Autodesk Inventor part; units mm, degrees
ref_plane "YZ Plane" through (0, 0, 0) normal (1, 0, 0) x (0, 1, 0)
ref_plane "XZ Plane" through (0, 0, 0) normal (0, 1, 0) x (-1, 0, 0)
ref_plane "XY Plane" through (0, 0, 0) normal (0, 0, 1) x (1, 0, 0)
sketch "Sketch1" plane through (0, 0, 0) normal (0, 0, 1) x (1, 0, 0)
  line L0 (-79.375, 79.375) -> (79.375, 79.375)
  line L1 (79.375, 79.375) -> (79.375, -79.375)
  line L2 (79.375, -79.375) -> (-79.375, -79.375)
  line L3 (-79.375, -79.375) -> (-79.375, 79.375)
  line L4 (-79.375, 79.375) -> (79.375, -79.375) construction
  line L5 (79.375, 79.375) -> (-79.375, -79.375) construction
  point P0 (0, 0)
  dimension "d0" = 158.75
extrude "Extrusion1" add sketch "Sketch1" along normal blind 50.8
shell "Shell1" thickness 3.175 outward yes removed faces 1 at (-26.4583, 26.4583, 50.8)
sketch "Sketch2" plane through (0, 0, 0) normal (0, 0, 1) x (1, 0, 0)
  line L0 (-82.55, 82.55) -> (-82.55, -82.55)
  circle A0 centre (-82.55, 82.55) radius 4.7752
  line L1 (82.55, -82.55) -> (82.55, 82.55)
  circle A1 centre (82.55, 82.55) radius 4.7752
  line L2 (-82.55, -82.55) -> (82.55, -82.55)
  circle A2 centre (82.55, -82.55) radius 4.7752
  circle A3 centre (-82.55, -82.55) radius 4.7752
  point P0 (0, 0)
  dimension "d4" = 9.5504
extrude "Extrusion2" add sketch "Sketch2" along normal blind 50.8 and the other way blind 3.175
sketch "Sketch3" plane through (0, 0, 50.8) normal (0, 0, 1) x (1, 0, 0)
  line L0 (-82.55, 77.7748) -> (-82.55, -77.7748)
  circle A0 centre (-82.55, -82.55) radius 1.7996
  circle A1 centre (82.55, 82.55) radius 1.7996
  line L1 (-77.7748, -82.55) -> (77.7748, -82.55)
  circle A2 centre (82.55, -82.55) radius 1.7996
  circle A3 centre (-82.55, 82.55) radius 1.7996
  point P0 (0, 0)
  dimension "d9" = 3.5992
extrude "Extrusion3" cut sketch "Sketch3" along normal mid plane 107.95
sketch "Sketch4" plane through (-77.7748, 82.55, -3.175) normal (0, 1, 0) x (1, 0, 0)
  line L0 (58.7248, -19.939) -> (96.8248, -19.939)
  line L1 (96.8248, -19.939) -> (96.8248, -42.545)
  line L2 (96.8248, -42.545) -> (58.7248, -42.545)
  line L3 (58.7248, -42.545) -> (58.7248, -19.939)
  line L4 (58.7248, -19.939) -> (96.8248, -42.545) construction
  line L5 (96.8248, -19.939) -> (58.7248, -42.545) construction
  line L6 (155.5496, -53.975) -> (0, -53.975)
  point P0 (77.7748, -3.175)
  point P1 (77.7748, -31.242)
  point P2 (77.7748, -31.242)
  point P3 (160.9128, -53.975)
  point P4 (-0.588, -53.975)
  dimension "d12" = 38.1
  dimension "d13" = 22.606
  dimension "d14" = 11.43
extrude "Extrusion4" cut sketch "Sketch4" against normal up to next
properties part number "PS-01" material "Aluminum 6061(1)"
Part model, mm, in its own coordinate system. A direction names the side the tool comes from. Coordinates: 2 decimals unless noted, no trailing zeros. Order: outer loops, then holes, each group sorted by start corner. A loop starts at its lowest first (then second) coordinate and runs counter-clockwise, first axis right, second up. Notation, with made-up numbers: (36.25, 66) - (58.25, 66) arc R33 ccw to (58.25, 102) - close; hole circle Ø1 at (18, 67). An arc over 180 degrees is marked (long way). Return JSON: item names as keys, results as strings. Group by question number.
Item 1: Cut at C-C (y = -10.5). List the corners of the cut face in (x, z) (3 decimals).
Item 2: Cut at A-A (x = 7). List the corners of the cut face in (y, z) (3 decimals), plus the area to 3 significant figures.
Item 3: Which spindle directions (+Z, -Z, +X, -X, +Y, -Y) get a long thin tool onto all of the face, cutting with end or side? Do faces 5 (the face through (-79.375, -1, 25)), 6 (the face through (1, -82.55, 23)), 7 (the face through (85.81, -86.04, 24.19)). Say none if no direction does.
Item 4: Cut at B-B (z = 43). List the corners of the cut face in (x, y) (3 decimals), plus the area to 3 significant figures.
Item 5: Pull direction X, two halves, no side cores. Call faces 1 (the face through (82.55, 1, 23)), 2 (the face through (-82.55, -1, 23)), 3 (the face through (-1, 1, -3.175)), 4 (the face through (-1, 82.55, 11)): pulls with the +X half, pulls with the -X half, needs draft (parallel to the pull), parting line crosses it, or undercut.
Item 6: Drill centre lines: probe 1 along X at (y, z) = (-68.5, 22.5) (3 decimals); probe 2 along Y at (x, z) = (-82, 15). Where is each one in solid material? Low to high. Write a range as from..to.
Item 7: Pin check, flat tips, straight feed: pin 1 (4 mm diameter, centred on x = -61, z = 42, fed in from +Y); pin 2 (4 mm diameter, centred on y = 49, z = 23, fed in from +X); pin 3 (6 mm diameter, centred on x = 82.55, y = 82.55, fed in from -Z) (3 decimals); pin 4 (1.5 mm diameter, centred on x = 57, y = 19.5, fed in from +Z). Stop position of each tip, or through.
Check values:
{
 "1": {"outline": "(-82.55, -3.175) - (82.55, -3.175) - (82.55, 50.8) - (79.375, 50.8) - (79.375, 0) - (-79.375, 0) - (-79.375, 50.8) - (-82.55, 50.8) - close"},
 "2": {"outline": "(-82.55, -3.175) - (82.55, -3.175) - (82.55, 16.764) - (79.375, 16.764) - (79.375, 0) - (-79.375, 0) - (-79.375, 50.8) - (-82.55, 50.8) - close; (79.375, 39.37) - (82.55, 39.37) - (82.55, 50.8) - (79.375, 50.8) - close", "area": "775 mm2"},
 "3": {"face 5": "+Z", "face 6": "+Z, -Z, -Y", "face 7": "+Z, -Z"},
 "4": {"outline": "(-82.55, -77.775) arc R4.775 ccw (long way) to (-77.775, -82.55) - (77.775, -82.55) arc R4.775 ccw (long way) to (82.55, -77.775) - (82.55, 77.775) arc R4.775 ccw (long way) to (77.775, 82.55) - (-77.775, 82.55) arc R4.775 ccw (long way) to (-82.55, 77.775) - close; hole circle Ø3.599 at (-82.55, -82.55); hole circle Ø3.599 at (-82.55, 82.55); hole (-79.375, -78.983) arc R4.775 cw to (-78.983, -79.375) - (78.983, -79.375) arc R4.775 cw to (79.375, -78.983) - (79.375, 78.983) arc R4.775 cw to (78.983, 79.375) - (-78.983, 79.375) arc R4.775 cw to (-79.375, 78.983) - close; hole circle Ø3.599 at (82.55, -82.55); hole circle Ø3.599 at (82.55, 82.55)", "area": "2,230 mm2"},
 "5": {"face 1": "pulls with the +X half", "face 2": "pulls with the -X half", "face 3": "needs draft", "face 4": "undercut"},
 "6": {"probe 1": "x = -82.55..-79.375, 79.375..82.55", "probe 2": "y = -87.29..-84.26, -80.84..80.84, 84.26..87.29"},
 "7": {"pin 1": "stops at y = 82.55", "pin 2": "stops at x = 82.55", "pin 3": "stops at z = -3.175", "pin 4": "stops at z = 0"}
}
